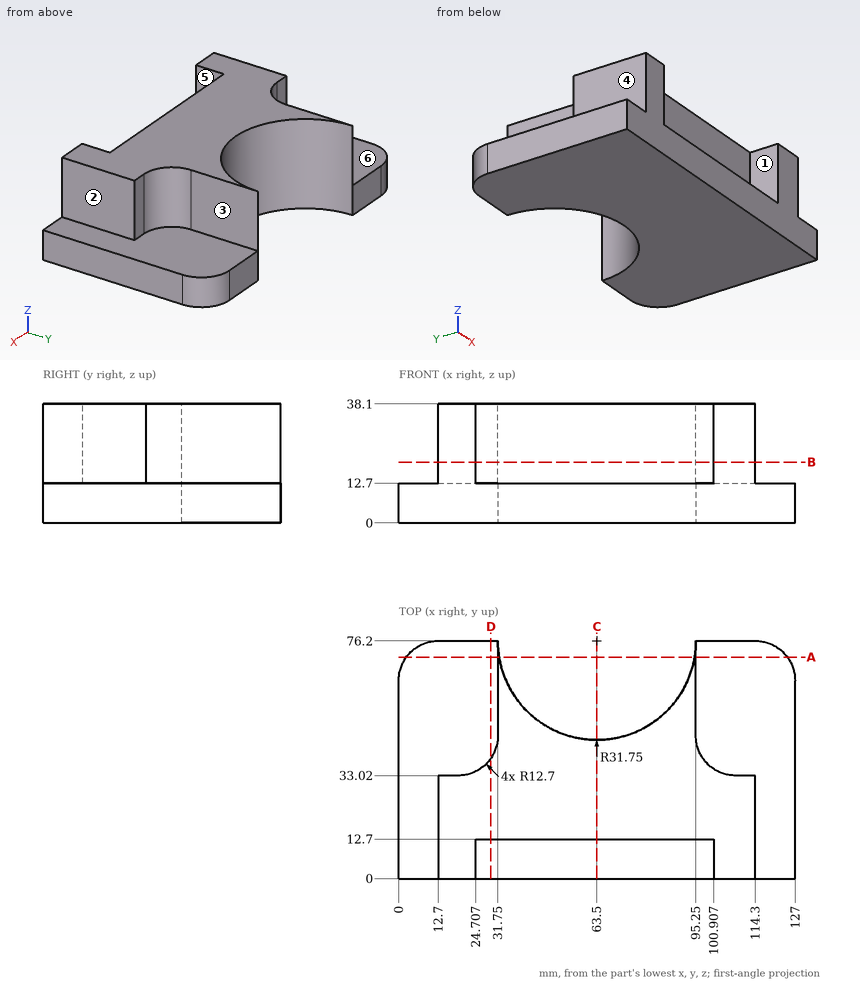
The drawing under review shows one solid part. Ordinate dimensions are in mm from its lowest x, y, z. A direction names the side the tool comes from. Round coordinates to 2 decimals unless told otherwise and drop trailing zeros. Write each loop counter-clockwise with the first axis right and the second up, starting at its lowest first coordinate (ties: lowest second). Pieces come first, ordered by that corner, then holes. Notation, with made-up numbers: (-3.5, 26.5) - (8.5, 26.5) arc R29 ccw to (8.5, 55.5) - close; hole circle Ø11 at (-9, 70.25). An arc over 180 degrees is marked (long way). Use a Markdown table: item, result. Add a question column.
1. We need section B-B (z = 19.5). State the section outline as (x, y) points.
2. Wall thickness on probe 1 along X at (y, z) = (12.5, 16); probe 2 along Z at (x, y) = (90, 5.5); probe 3 along X at (y, z) = (15, 20): over which ranges is each line inside the solid? List them lowest first.
3. For the marked faces 1, 2 and 3, list the 3-axis set-ups (+Z, -Z, +X, -X, +Y, -Y) from which the entire face can be reached by the end or side of a thin tool; tool diameter is ignored.
4. We need section C-C (x = 63.5). State the section outline as (y, z) points, then the cut area to 3 significant figures.
5. We need section D-D (x = 29.5). State the section outline as (y, z) points.
6. Clearance check with flat-ended pins moving along their axes: pin 1 (2 mm diameter, centred on y = 62, z = 33.5, fed in from -X); pin 2 (6.5 mm diameter, centred on x = 70.5, y = 5, fed in from +Z); pin 3 (14 mm diameter, centred on y = 7.5, z = 22.5, fed in from +X). State where each tip first meets the part, or that it passes through.
7. Mouldability with a two-part tool opening along X and no side actions: class the marked faces 4, 5 and 6 as +X half, -X half, draft (parallel to the pull), parting line (faces both ways), or undercut.
8. We need section A-A (y = 71). State the section outline as (x, z) points, then the cut area to 3 significant figures.
Output:
| question | item | result |
|---|---|---|
| 1 | outline | (12.7, 0) - (24.71, 0) - (24.71, 12.7) - (100.91, 12.7) - (100.91, 0) - (114.3, 0) - (114.3, 33.02) - (107.95, 33.02) arc R12.7 cw to (95.25, 45.72) - (95.25, 76.2) arc R31.75 cw to (31.75, 76.2) - (31.75, 45.72) arc R12.7 cw to (19.05, 33.02) - (12.7, 33.02) - close |
| 2 | probe 1 | x = 12.7 to 24.71, 100.91 to 114.3 |
| 2 | probe 2 | z = 0 to 12.7 |
| 2 | probe 3 | x = 12.7 to 114.3 |
| 3 | face 1 | +Z, -Y |
| 3 | face 2 | +Z, +X, +Y, -Y |
| 3 | face 3 | +Z, +X, +Y |
| 4 | outline | (0, 0) - (44.45, 0) - (44.45, 38.1) - (12.7, 38.1) - (12.7, 12.7) - (0, 12.7) - close |
| 4 | area | 1,370 mm2 |
| 5 | outline | (0, 0) - (76.2, 0) - (76.2, 12.7) - (38.5, 12.7) - (38.5, 38.1) - (12.7, 38.1) - (12.7, 12.7) - (0, 12.7) - close |
| 6 | pin 1 | stops at x = 31.75 |
| 6 | pin 2 | stops at z = 12.7 |
| 6 | pin 3 | stops at x = 114.3 |
| 7 | face 4 | -X half |
| 7 | face 5 | undercut |
| 7 | face 6 | draft |
| 8 | outline | (2.45, 0) - (32.18, 0) - (32.18, 38.1) - (31.75, 38.1) - (31.75, 12.7) - (2.45, 12.7) - close; (94.82, 0) - (124.55, 0) - (124.55, 12.7) - (95.25, 12.7) - (95.25, 38.1) - (94.82, 38.1) - close |
| 8 | area | 777 mm2 |
